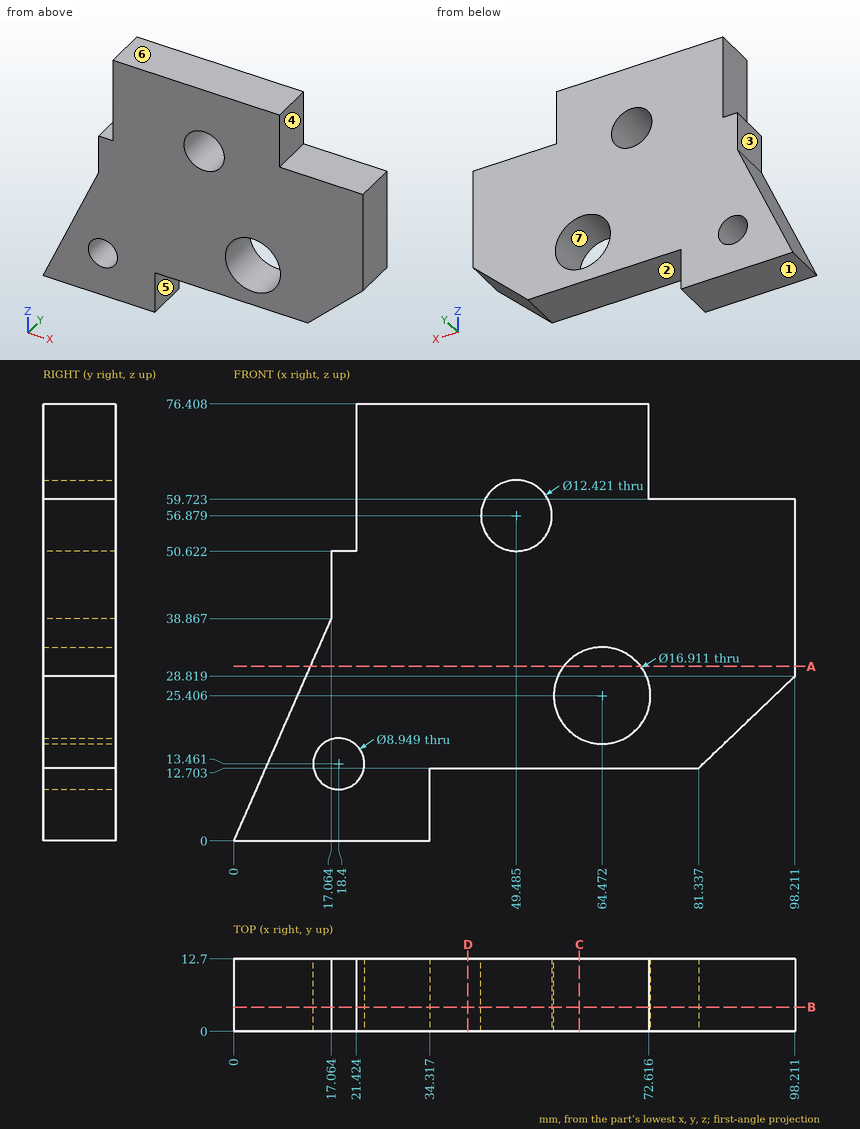
Study the drawing (mm; zero at the part's minimum x, y, z) and answer. A direction names the side the tool comes from. Give positions to 0.01 mm unless a question says otherwise; leave off trailing zeros. Write each loop counter-clockwise with the first axis right and the second up, starting at its lowest first coordinate (ties: lowest second). Pieces come first, ordered by that corner, then holes. Notation, with made-up numbers: (16.25, -13) -> (42.25, -13) arc R19 ccw to (42.25, 3) -> close; hole circle Ø4 at (-19, 5). An arc over 180 degrees is marked (long way). Write item = value, one per line. Start each with the question number.
1) The part is cut by section B-B, the plane y = 4.25. Count the separate pieces of the cut face and the enclosed holes in it, and give its area (3 significant figures).
2) Each of these flat-tipped pins is pushed along its axis until it touches: pin 1 (2 mm diameter, centred on x = 48.5, y = 4.5, fed in from -Z); pin 2 (1.3 mm diameter, centred on x = 20, y = 9.5, fed in from +Z); pin 3 (5 mm diameter, centred on y = 3.5, z = 17.5, fed in from -X) (1 decimal). Where does it stop, or does it pass through?
3) The part is cut by section C-C, the plane x = 60.5. Determine the outline of the cut face in (y, z).
4) Which of the six approach directions +Z, -Z, +X, -X, +Y, -Y give full straight-line access (tool end or side, diameter ignored) to the marked faces 1, 2, 3 and 4?
5) Straight lines are drawn through the part: line 1 along Z through (x, y) = (76, 9); line 2 along Z through (x, y) = (37, 8.5); line 3 along X through (y, z) = (9.5, 73) (1 decimal). For each, find the intervals that lie inside material, in ascending order.
6) The part is cut by section D-D, the plane x = 41. Determine the outline of the cut face in (y, z), and give its area (3 significant figures).
7) The part is cut by section A-A, the plane z = 30.5. Determine the outline of the cut face in (x, y), and give its area (3 significant figures).
8) Determine the mould class of the marked faces 5, 6 and 7 for opening direction X: +X half, -X half, draft (parallel to the pull), parting line (faces both ways), or undercut.
Solutions:
q1.separate_pieces = 1
q1.enclosed_holes = 3
q1.area = 4,640 mm²
q2.pin_1 = 12.7
q2.pin_2 = 50.62
q2.pin_3 = 6.6
q3.outline = (0, 12.7) -> (12.7, 12.7) -> (12.7, 17.94) -> (0, 17.94) -> close; (0, 32.87) -> (12.7, 32.87) -> (12.7, 76.41) -> (0, 76.41) -> close
q4.face_1 = -Z, +X, -X, +Y, -Y
q4.face_2 = -Z, +X, +Y, -Y
q4.face_3 = +Z, -X, +Y, -Y
q4.face_4 = +Z, +X, +Y, -Y
q5.line_1 = 12.7 to 59.72
q5.line_2 = 12.7 to 76.41
q5.line_3 = 21.4 to 72.6
q6.outline = (0, 12.7) -> (12.7, 12.7) -> (12.7, 76.41) -> (0, 76.41) -> close
q6.area = 809 mm²
q7.outline = (13.39, 0) -> (57.72, 0) -> (57.72, 12.7) -> (13.39, 12.7) -> close; (71.22, 0) -> (98.21, 0) -> (98.21, 12.7) -> (71.22, 12.7) -> close
q7.area = 906 mm²
q8.face_5 = +X half
q8.face_6 = draft
q8.face_7 = undercut
